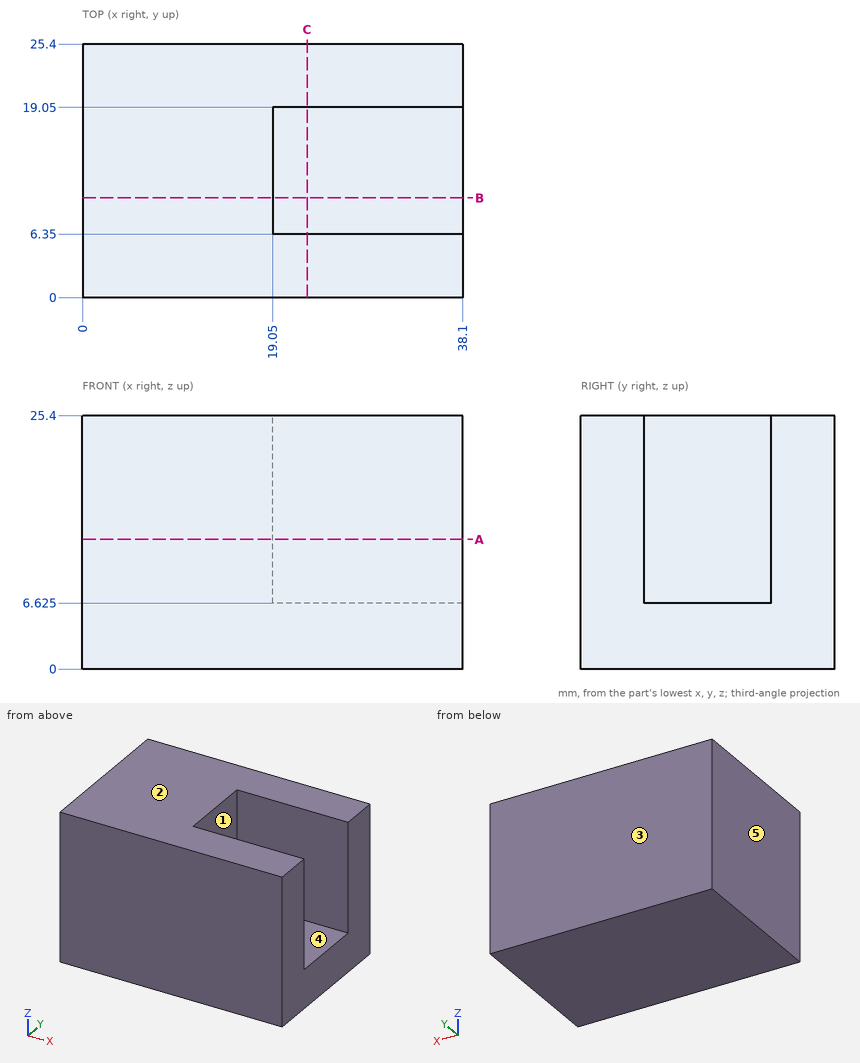
Can you work these out from the drawing? Everything is in mm from the part's minimum corner. A direction names the side the tool comes from. Coordinates: 2 decimals unless noted, no trailing zeros. Write each loop counter-clockwise with the first axis right and the second up, starting at its lowest first coordinate (ties: lowest second). Pieces come first, ordered by that corner, then holes. Notation, with made-up numbers: (20, 43.5) -> (24, 43.5) arc R18 ccw to (24, 75.5) -> close; hole circle Ø7 at (-32, 73.25). An arc over 180 degrees is marked (long way). Write each question's results on one line, items separated by ' | '. Start each with the question number.
Q1. I'm going to push flat-ended pins straight in: pin 1 (4 mm diameter, centred on x = 29, y = 13, fed in from +Z) (3 decimals); pin 2 (10 mm diameter, centred on y = 13, z = 13.5, fed in from +X). Where does each tip first touch, or does it pass through?
Q2. We'd pull the mould along Y, two halves only. Please class the marked faces 3, 4 and 5: +Y half, -Y half, draft (parallel to the pull), parting line (faces both ways), or undercut.
Q3. Imagine slicing it at C-C (x = 22.5). Write out the boundary of the cut face in (y, z) (3 decimals), then the cut area to 3 significant figures.
Q4. If I drill on probe 1 along Y at (x, z) = (29.5, 14.75); probe 2 along Z at (x, y) = (24, 13.25) (3 decimals); probe 3 along X at (y, z) = (11.5, 22.75), over which ranges is the centre line in solid material (lowest first)?
Q5. Imagine slicing it at B-B (y = 10). Write out the boundary of the cut face in (x, z) (3 decimals).
Q6. Imagine slicing it at A-A (z = 13). Write out the boundary of the cut face in (x, y), then the cut area to 3 significant figures.
Q7. On a 3-axis mill with a long thin cutter (end or side, diameter ignored), from which of +Z, -Z, +X, -X, +Y, -Y can I reach the whole of each face in a straight line? I mean the marked faces 1 and 2. Say none if no direction works.
Taken from the geometry:
1) pin 1: stops at z = 6.625 | pin 2: stops at x = 19.05
2) face 3: +Y half | face 4: undercut | face 5: draft
3) outline: (0, 0) -> (25.4, 0) -> (25.4, 25.4) -> (19.05, 25.4) -> (19.05, 6.625) -> (6.35, 6.625) -> (6.35, 25.4) -> (0, 25.4) -> close | area: 407 mm^2
4) probe 1: y = 0 to 6.35, 19.05 to 25.4 | probe 2: z = 0 to 6.625 | probe 3: x = 0 to 19.05
5) outline: (0, 0) -> (38.1, 0) -> (38.1, 6.625) -> (19.05, 6.625) -> (19.05, 25.4) -> (0, 25.4) -> close
6) outline: (0, 0) -> (38.1, 0) -> (38.1, 6.35) -> (19.05, 6.35) -> (19.05, 19.05) -> (38.1, 19.05) -> (38.1, 25.4) -> (0, 25.4) -> close | area: 726 mm^2
7) face 1: +Z, +X | face 2: +Z, +X, -X, +Y, -Y
